The listing builds one solid part. Answer for the finished solid, in the listing's coordinates (mm). A direction names the side the tool comes from. Round coordinates to 2 decimals unless told otherwise and drop trailing zeros. Loops run counter-clockwise (first coordinate to the right, second up) from the corner with the lowest first, then second, coordinate; pieces in that order, holes last. Notation, with made-up numbers: (11, -39) - (44, -39) arc R13 ccw to (44, -26) - close; hole circle Ø7 at (79.25, 45). An arc over 180 degrees is marked (long way). One line per item, written item: value.
Autodesk Inventor part; units mm, degrees
ref_plane "Work Plane3" through (238.7196, -108.8102, 126.4793) normal (0, 0, -1) x (0, 1, 0)
ref_plane "YZ Plane" through (0, 0, 0) normal (1, 0, 0) x (0, 1, 0)
ref_plane "XZ Plane" through (0, 0, 0) normal (0, 1, 0) x (-1, 0, 0)
sketch "Sketch1" plane through (0, 0, 0) normal (0, 0, 1) x (1, 0, 0)
  line L0 (-63.5719, 111.8382) -> (-7.6155, -96.5129) construction
  line L1 (-12.4444, -97.8098) -> (-68.7777, 111.945) construction
  line L2 (-42.0741, -26.0387) -> (-40.7772, -30.8676)
  line L3 (-40.7772, -30.8676) -> (304.995, 61.9956)
  line L4 (304.995, 61.9956) -> (303.6981, 66.8245)
  line L5 (-23.1781, -38.5663) -> (-40.7772, -30.8676) construction
  line L6 (247.1858, -96.9584) -> (307.8088, 111.597) construction
  line L7 (-42.0741, -26.0387) -> (-32.4163, -23.445) construction
  line L8 (294.0403, 64.2307) -> (303.6981, 66.8245) construction
  line L9 (-42.0741, -26.0387) -> (303.6981, 66.8245)
  point P0 (0, 0)
extrude "Extrusion1" add sketch "Sketch1" along normal blind 100
ref_plane "Work Plane1" through (0, 0, 50) normal (0, 0, 1) x (1, 0, 0)
sketch "Sketch3" plane through (0, 0, 100) normal (0, 0, 1) x (1, 0, 0)
  line L0 (302.6018, 111.597) -> (307.8088, 111.597) construction
  line L1 (302.6018, 111.597) -> (242.3845, -95.5627) construction
  line L2 (242.3845, -95.5627) -> (247.1858, -96.9584) construction
  line L3 (247.1858, -96.9584) -> (307.8088, 111.597) construction
  line L4 (-42.0741, -26.0387) -> (-40.7772, -30.8676) construction
  line L5 (-40.7772, -30.8676) -> (304.995, 61.9956) construction
  line L6 (304.995, 61.9956) -> (303.6981, 66.8245) construction
  line L7 (303.6981, 66.8245) -> (-42.0741, -26.0387) construction
  line L8 (285.4632, 61.9272) -> (286.7601, 57.0983)
  line L9 (286.7601, 57.0983) -> (295.3372, 59.4019)
  line L10 (295.3372, 59.4019) -> (294.0403, 64.2307)
  line L11 (294.0403, 64.2307) -> (285.4632, 61.9272)
  point P0 (0, 0)
extrude "Extrusion2" cut sketch "Sketch3" against normal up to surface (50 mm away)
sketch "Sketch4" plane through (0, 0, 100) normal (0, 0, 1) x (1, 0, 0)
  line L0 (286.7601, 57.0983) -> (285.4632, 61.9272) construction
  line L1 (285.4632, 61.9272) -> (-42.0741, -26.0387) construction
  line L2 (-42.0741, -26.0387) -> (-40.7772, -30.8676) construction
  line L3 (-40.7772, -30.8676) -> (286.7601, 57.0983) construction
  line L4 (-63.5719, 111.8382) -> (-68.7777, 111.945) construction
  line L5 (-12.4444, -97.8098) -> (-68.7777, 111.945) construction
  line L6 (-7.6155, -96.5129) -> (-12.4444, -97.8098) construction
  line L7 (-63.5719, 111.8382) -> (-7.6155, -96.5129) construction
  line L8 (-40.7772, -30.8676) -> (286.7601, 57.0983) construction
  line L9 (-32.4163, -23.445) -> (-31.1195, -28.2739)
  line L10 (-31.1195, -28.2739) -> (-26.2906, -26.977)
  line L11 (-26.2906, -26.977) -> (-27.5875, -22.1481)
  line L12 (-27.5875, -22.1481) -> (-32.4163, -23.445)
  line L13 (-32.6578, -23.5098) -> (-31.3609, -28.3387)
  line L14 (-31.3609, -28.3387) -> (-26.0491, -26.9121)
  line L15 (-26.0491, -26.9121) -> (-27.346, -22.0832)
  line L16 (-27.346, -22.0832) -> (-32.6578, -23.5098)
  line L17 (285.4632, 61.9272) -> (-42.0741, -26.0387)
  point P0 (0, 0)
  point P1 (-28.705, -27.6254)
  dimension "d21" = 5.5
extrude "Extrusion3" cut sketch "Sketch4" against normal up to surface (50 mm away)
ref_plane "Work Plane2" through (315.6821, 138.6828, 40.9) normal (0.0484699, 0.1667464, -0.9848078) x (-0.9602541, 0.2791272, 0)
ref_plane "Work Plane3" through (238.7196, -108.8102, 126.4793) normal (0, 0, -1) x (0, 1, 0)
sketch "Sketch6" plane through (303.6981, 66.8245, 100) normal (-0.2593763, 0.9657763, 0) x (0.9657763, 0.2593763, 0)
  line L0 (-348.2751, 50) -> (-342.7751, 50) construction
  line L1 (-18.881, 0) -> (-342.7751, 0) construction
  line L2 (-18.881, 0) -> (-18.881, 50) construction
  line L3 (-18.881, 50) -> (-10, 50) construction
  line L4 (-10, 50) -> (-10, 0) construction
  line L5 (0, 0) -> (-10, 0) construction
  line L6 (0, 100) -> (0, 0) construction
  line L7 (0, 100) -> (-358.0251, 100) construction
  line L8 (-358.0251, 100) -> (-358.0251, 0) construction
  line L9 (-14.0857, 72.7069) -> (0, 72.7069)
  line L10 (0, 100) -> (0, 0) construction
  line L11 (0, 72.7069) -> (0, 100)
  line L12 (-358.0251, 100) -> (0, 100)
  line L13 (0, 100) -> (-358.0251, 100)
  line L14 (-358.0251, 100) -> (-358.0251, 88.8925)
  line L15 (-358.0251, 100) -> (-358.0251, 0) construction
  line L16 (-343.0251, 88.8925) -> (-358.0251, 88.8925)
  line L17 (-343.0251, 88.8925) -> (-14.0857, 72.7069)
  line L18 (-358.0251, 100) -> (-358.0251, 0) construction
  line L19 (-342.7751, 50) -> (-342.7751, 0)
  line L20 (-348.2751, 0) -> (-358.0251, 0)
  line L21 (-348.2751, 0) -> (-348.2751, 50)
  point P0 (-310.6371, 100)
extrude "Extrusion5" cut sketch "Sketch6" against normal through all
sketch "Sketch7" plane through (285.4632, 61.9272, 100) normal (-0.2593763, 0.9657763, 0) x (0.9657763, 0.2593763, 0)
  line L0 (18.881, 72.7069) -> (18.881, 0) construction
  line L1 (-339.1441, 88.8925) -> (-339.1441, 0) construction
  line L2 (-323.8941, 4.5) -> (-339.1441, 4.5)
  line L3 (-339.1441, 4.5) -> (-339.1441, 0)
  line L4 (-339.1441, 0) -> (18.881, 0)
  line L5 (-339.1441, 0) -> (18.881, 0)
  line L6 (8.881, 0) -> (18.881, 0)
  line L7 (18.881, 0) -> (18.881, 25)
  line L8 (0, 0) -> (0, 50) construction
  line L9 (18.881, 25) -> (0, 25)
  line L10 (0, 25) -> (-323.8941, 4.5)
  line L11 (0, 50) -> (8.881, 50) construction
  line L12 (-323.8941, 50) -> (-323.8941, 0) construction
  point P0 (-291.7561, 100)
  dimension "d17" = 25
  dimension "d18" = 4.5
ref_plane "Work Plane4" through (315.6821, 138.6828, 45.9) normal (0.9602541, -0.2791272, 0) x (0.2791272, 0.9602541, 0)
sketch "Sketch8" plane through (315.6821, 138.6828, 45.9) normal (0.9602541, -0.2791272, 0) x (0.2791272, 0.9602541, 0)
  line L0 (-245.3946, 71.5637) -> (-28.2069, 15.6815) construction
  line L1 (-82.1398, 54.1) -> (-82.1398, 4.1) construction
  point P0 (-221.2862, -45.9)
  point P1 (-82.1398, 29.5584)
  dimension "d16" = 25.4584
ref_plane "Work Plane5" through (-76.0939, 139.1865, 45.8) normal (-0.9657763, -0.2593763, 0) x (-0.2593763, 0.9657763, 0)
extrude "Extrusion6" cut sketch "Sketch7" against normal through all
properties part number "brace"
1) A cutting plane is placed at A-A on z = 89. Give the vertices of the cut face in (x, y), and give its area (3 significant figures).
Final values:
outline: (-42.07, -26.04) - (-40.78, -30.87) - (-31.36, -28.34) - (-32.66, -23.51) - close; (-27.35, -22.08) - (-26.05, -26.91) - (73.13, -0.27) - (71.84, 4.55) - close
area: 562 mm2
2) For faces 4 (the flat face through (300, 63, 75)), 5 (the flat face through (297, 63, 27.293)), determine the directions among +Z, -Z, +X, -X, +Y, -Y from which every point of the face is accessible in a straight line to the end or side of a thin tool.
Final values:
face 4: +Z, +X, +Y, -Y
face 5: -Z, +X, +Y, -Y
3) Each of these flat-tipped pins is pushed along its axis until it touches: pin 1 Ø6 at (x, y) = (71.5, 2.5) entering from -Z; pin 2 Ø8 at (x, y) = (299.5, 64.5) entering from +Z; pin 3 Ø2.5 at (x, y) = (298.5, 63) entering from -Z. Where does it stop, or does it pass through?
Final values:
pin 1: z = 15.98
pin 2: z = 75
pin 3: z = 27.29
4) Consider L1, parallel to Y at x = 226.5, z = 38.5; L2, parallel to Y at x = 190, z = 71.5; L3, parallel to Z at x = 243, y = 50. Determine where each line is inside the solid, lowest interval first.
Final values:
L1: 40.91 to 46.09
L2: 31.11 to 36.29
L3: 24.89 to 77.79
5) A cutting plane is placed at D-D on x = 172. Give the vertices of the cut face in (y, z).
Final values:
outline: (26.28, 21.21) - (31.45, 21.28) - (31.45, 82.44) - (26.28, 82.52) - close
6) A cutting plane is placed at B-B on z = 57. Give the vertices of the cut face in (x, y) (1 decimal), and give its area (3 significant figures).
Final values:
outline: (-42.1, -26) - (-40.8, -30.9) - (-31.4, -28.3) - (-32.7, -23.5) - close; (-27.3, -22.1) - (-26, -26.9) - (286.8, 57.1) - (285.5, 61.9) - close; (294, 64.2) - (295.3, 59.4) - (305, 62) - (303.7, 66.8) - close
area: 1,720 mm2
7) For a pull along X with two mould halves and no side action, classify faces 1 (the flat face through (290, 61, 50)), 2 (the flat face through (89.972, 9.425, 52.713)), 3 (the flat face through (-34, -26, 11.108)) as released by +X, released by -X, zero draft, split by the parting line, or undercut.
Final values:
face 1: undercut
face 2: released by -X
face 3: zero draft
8) A cutting plane is placed at C-C on y = -11. Give the vertices of the cut face in (x, z).
Final values:
outline: (13.92, 13.22) - (33.2, 14.14) - (33.2, 91.62) - (13.92, 92.8) - close
